Geometry: final body of the model. Coordinates: model frame, mm. Face numbers are marked on the shaded views. Give positions to 0.01 mm unless a question says otherwise; leave off trailing zeros. Loops run counter-clockwise (first coordinate to the right, second up) from the corner with the lowest first, then second, coordinate; pieces in that order, holes last. Notation, with made-up numbers: (32, -15.5) -> (62, -15.5) arc R16 cw to (62, -5.5) -> close; hole circle Ø9 at (35, -11). An arc over 180 degrees is marked (long way). Answer in a Markdown table with one row per item. Add a question column.
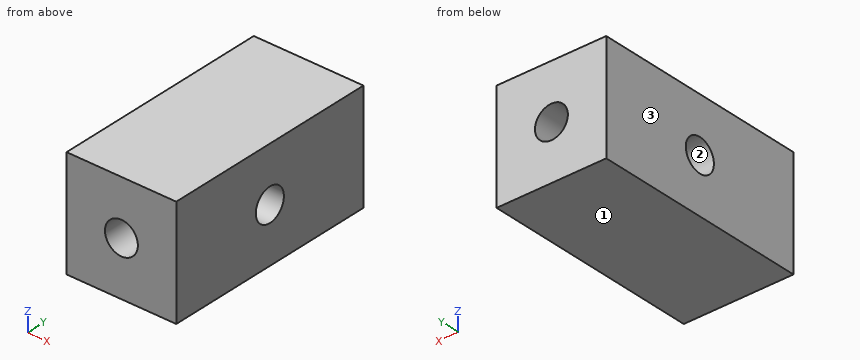
from build123d import *

# Parameters (mm, degrees)
SKETCH1_W           = 10
SKETCH1_H           = 10
BOSS_EXTRUDE1_DEPTH = 20
SKETCH4_R           = 1.5
CUT_EXTRUDE2_DEPTH  = 11
SKETCH5_R           = 1.5
CUT_EXTRUDE3_DEPTH  = 21


with BuildPart() as part:
    # Sketch1 → Boss-Extrude1 (new body)
    with BuildSketch(Plane(origin=(0, 0, 0), x_dir=(1, 0, 0), z_dir=(0, 1, 0))):
        Rectangle(SKETCH1_W, SKETCH1_H)
    extrude(amount=BOSS_EXTRUDE1_DEPTH)

    # Sketch4 → Cut-Extrude2 (cut, through all)
    with BuildSketch(Plane(origin=(5, 0, 0), x_dir=(0, 0, -1), z_dir=(1, 0, 0))):
        with Locations((0, 10)):
            Circle(SKETCH4_R)
    extrude(amount=-CUT_EXTRUDE2_DEPTH, mode=Mode.SUBTRACT)

    # Sketch5 → Cut-Extrude3 (cut, through all)
    with BuildSketch(Plane(origin=(0, 20, 0), x_dir=(1, 0, 0), z_dir=(0, 1, 0))):
        Circle(SKETCH5_R)
    extrude(amount=-CUT_EXTRUDE3_DEPTH, mode=Mode.SUBTRACT)


solid = part.part
(1) Pin query (flat end, axial travel): pin 1 Ø4 at (x, z) = (0, 0) entering from -Y. Return the tip coordinate at first contact, or that it passes through.
(2) Cut plane B-B on x = -0.5. Return the cut outline in (y, z).
(3) Draft query along Z for the marked faces 1, 2 and 3. Return one class per face: +Z half, -Z half, draft (parallel to the pull), parting line (faces both ways), or undercut.
(4) Cut plane C-C on y = 4. Return the cut outline in (x, z), then the cut area to 3 significant figures.
(5) Cut plane D-D on x = -3.5. Return the cut outline in (y, z), then the cut area to 3 significant figures.
(6) Material intervals for line 1 along Z through (x, y) = (-2.05, 10); line 2 along Y through (x, z) = (2.4, 0), sorted ascending. Write a range as from..to.
(7) Cut plane A-A on z = 0. Return the cut outline in (x, y), then the cut area to 3 significant figures.
Answer list:
| question | item | result |
|---|---|---|
| 1 | pin 1 | stops at y = 0 |
| 2 | outline | (0, -5) -> (20, -5) -> (20, -1.41) -> (10.5, -1.41) arc R1.5 cw to (9.5, -1.41) -> (0, -1.41) -> close; (0, 1.41) -> (9.5, 1.41) arc R1.5 cw to (10.5, 1.41) -> (20, 1.41) -> (20, 5) -> (0, 5) -> close |
| 3 | face 1 | -Z half |
| 3 | face 2 | undercut |
| 3 | face 3 | draft |
| 4 | outline | (-5, -5) -> (5, -5) -> (5, 5) -> (-5, 5) -> close; hole circle Ø3 at (0, 0) |
| 4 | area | 92.9 mm² |
| 5 | outline | (0, -5) -> (20, -5) -> (20, 5) -> (0, 5) -> close; hole circle Ø3 at (10, 0) |
| 5 | area | 193 mm² |
| 6 | line 1 | z = -5..-1.5, 1.5..5 |
| 6 | line 2 | y = 0..8.5, 11.5..20 |
| 7 | outline | (-5, 0) -> (-1.5, 0) -> (-1.5, 8.5) -> (-5, 8.5) -> close; (-5, 11.5) -> (-1.5, 11.5) -> (-1.5, 20) -> (-5, 20) -> close; (1.5, 0) -> (5, 0) -> (5, 8.5) -> (1.5, 8.5) -> close; (1.5, 11.5) -> (5, 11.5) -> (5, 20) -> (1.5, 20) -> close |
| 7 | area | 119 mm² |
